```python
from build123d import *

# Parameters (mm, degrees)
BOSS_EXTRU_1_DEPTH      = 18
ESQUISSE2_W             = 12.72
ESQUISSE2_H             = 15
ENL_V_MAT_EXTRU_1_DEPTH = 12.7
ESQUISSE3_R             = 2.525
ENL_V_MAT_EXTRU_2_DEPTH = 27


with BuildPart() as part:
    # Esquisse1 → Boss.-Extru.1 (new body)
    with BuildSketch(Plane.XY):
        with BuildLine():
            Line((0, 0), (26, 0))
            Line((26, 0), (26, 27))
            Line((26, 27), (23.5, 27))
            ThreePointArc((23.5, 27), (13, 20), (2.5, 27))
            Line((2.5, 27), (0, 27))
            Line((0, 27), (0, 0))
        make_face()
    extrude(amount=BOSS_EXTRU_1_DEPTH)

    # Esquisse2 → Enlèv. mat.-Extru.1 (cut)
    with BuildSketch(Plane.XY.offset(18)):
        with Locations((13, 7.5)):
            Rectangle(ESQUISSE2_W, ESQUISSE2_H)
    extrude(amount=-ENL_V_MAT_EXTRU_1_DEPTH, mode=Mode.SUBTRACT)

    # Esquisse3 → Enlèv. mat.-Extru.2 (cut, through all)
    with BuildSketch(Plane.ZY):
        with Locations((11.65, 7.13)):
            Circle(ESQUISSE3_R)
    extrude(amount=-ENL_V_MAT_EXTRU_2_DEPTH, mode=Mode.SUBTRACT)


solid = part.part
```
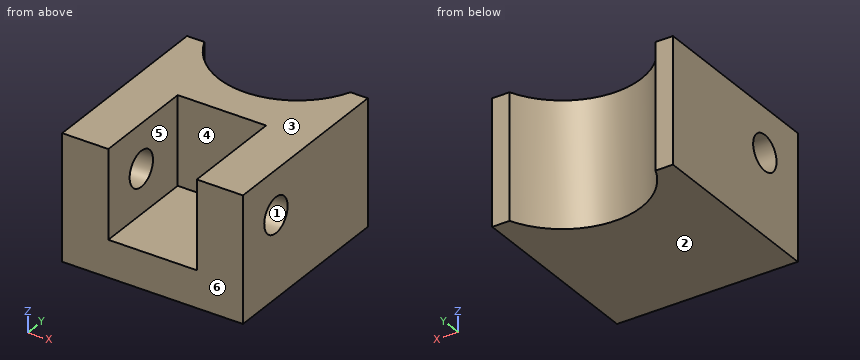
Geometry check sheet. Reference: the model listing, model coordinates, mm. Face numbers are marked on the shaded views. A direction names the side the tool comes from. Coordinates: 2 decimals unless noted, no trailing zeros. Write each loop counter-clockwise with the first axis right and the second up, starting at its lowest first coordinate (ties: lowest second). Pieces come first, ordered by that corner, then holes. Notation, with made-up numbers: M 75.25,-21.5 L 88.25,-21.5 A9 ccw 88.25,-4.5 Z; hole C 83,10.5 d11. An arc over 180 degrees is marked long. One line per item, written item: value. Start each with the question number.
(1) Sectioned sample at D-D, the plane x = 24. Enter the section's corners in (y, z) (3 decimals), and give its area (3 significant figures).
(2) Sectioned sample at C-C, the plane y = 7.13. Enter the section's corners in (x, z) (3 decimals).
(3) Sectioned sample at A-A, the plane z = 11.65. Enter the section's corners in (x, y) (3 decimals), and give its area (3 significant figures).
(4) Scan lines: line 1 along Y through (x, z) = (1.75, 11.65) (3 decimals); line 2 along X through (y, z) = (8, 8.25); line 3 along Z through (x, y) = (6.5, 7.75). Record each from-to range of solid material in increasing order. Write a range as [from, to].
(5) Sectioned sample at B-B, the plane y = 11.5. Enter the section's corners in (x, z).
(6) Release check for a two-part mould opening along Z. For the marked faces 1, 2, 3 and 4 record: released by +Z, released by -Z, zero draft, split by the parting line, or undercut.
(7) Tool access check on the marked faces 5 and 6. Record the directions out of +Z, -Z, +X, -X, +Y, -Y that give a thin tool (end or side, any length) a straight path to the whole face; none if there is none.
(8) Depth check by flat-ended pin: pin 1 (8 mm diameter, centred on x = 11.5, z = 11, fed in from -Y); pin 2 (1.5 mm diameter, centred on x = 18.5, z = 4.5, fed in from +Y). Enter the tip coordinate at first touch or a pass-through.
Filled sheet:
1. outline: M 0,0 L 27,0 L 27,18 L 0,18 Z; hole C 7.13,11.65 d5.05
1. area: 466 mm²
2. outline: M 0,0 L 26,0 L 26,9.125 L 19.36,9.125 L 19.36,5.3 L 6.64,5.3 L 6.64,9.125 L 0,9.125 Z; M 0,14.175 L 6.64,14.175 L 6.64,18 L 0,18 Z; M 19.36,14.175 L 26,14.175 L 26,18 L 19.36,18 Z
3. outline: M 0,0 L 6.64,0 L 6.64,4.605 L 0,4.605 Z; M 0,9.655 L 6.64,9.655 L 6.64,15 L 19.36,15 L 19.36,9.655 L 26,9.655 L 26,27 L 23.5,27 A11.375 cw 2.5,27 L 0,27 Z; M 19.36,0 L 26,0 L 26,4.605 L 19.36,4.605 Z
3. area: 338 mm²
4. line 1: [0, 4.605], [9.655, 27]
4. line 2: [0, 6.64], [19.36, 26]
4. line 3: [0, 9.2], [14.1, 18]
5. outline: M 0,0 L 26,0 L 26,18 L 19.36,18 L 19.36,5.3 L 6.64,5.3 L 6.64,18 L 0,18 Z
6. face 1: undercut
6. face 2: released by -Z
6. face 3: released by +Z
6. face 4: zero draft
7. face 5: +Z, -Y
7. face 6: +Z, -Z, +X, -X, -Y
8. pin 1: y = 15
8. pin 2: y = 21.87
